Part model, mm, in its own coordinate system. Face numbers are marked on the shaded views. A direction names the side the tool comes from. Coordinates: 2 decimals unless noted, no trailing zeros. Loops run counter-clockwise (first coordinate to the right, second up) from the corner with the lowest first, then second, coordinate; pieces in that order, holes last. Notation, with made-up numbers: M 44.25,-3 L 51.25,-3 A24 cw 51.25,16 Z; hole C -8,56 d8. An arc over 180 degrees is marked long. Use CSV: the item, a comma, the result in double quotes. Start each with the question number.
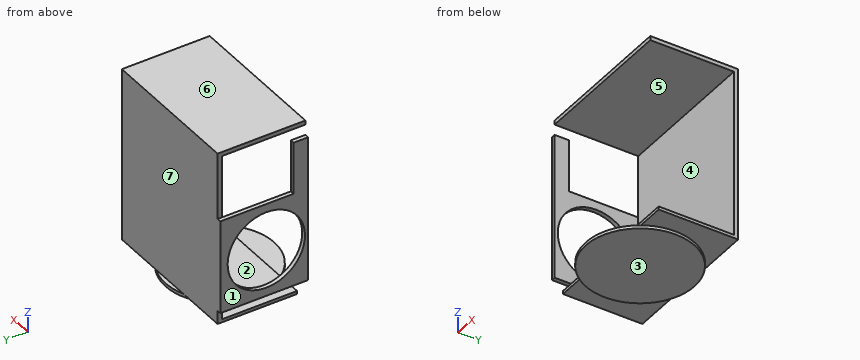
from build123d import *

# Parameters (mm, degrees)
SKETCH_1_R      = 26
EXTRUDE_1_DEPTH = 1.5
EXTRUDE_2_DEPTH = 1.5
SKETCH_3_W      = 70
SKETCH_3_H      = 2
EXTRUDE_3_DEPTH = 82
SKETCH_4_W      = 70
SKETCH_4_H      = 2
EXTRUDE_4_DEPTH = 40
SKETCH_5_R      = 18.5
EXTRUDE_5_DEPTH = 2


with BuildPart() as part:
    # 草图1 → 凸台-拉伸1 (new body)
    with BuildSketch(Plane.XY):
        Circle(SKETCH_1_R)
    extrude(amount=EXTRUDE_1_DEPTH)

    # 草图2 → 凸台-拉伸2 (add)
    with BuildSketch(Plane.XY.offset(1.5)):
        Polygon((-35, 24), (-35, -14), (-21.9089023, -14), (21.9089023, -14), (35, -14), (35, 24), align=None)
    extrude(amount=EXTRUDE_2_DEPTH)

    # 草图3 → 凸台-拉伸3 (add)
    with BuildSketch(Plane.XY.offset(3)):
        with Locations((0, 23)):
            Rectangle(SKETCH_3_W, SKETCH_3_H)
    extrude(amount=EXTRUDE_3_DEPTH)

    # 草图4 → 凸台-拉伸4 (add)
    with BuildSketch(Plane.XZ.offset(-22)):
        with Locations((0, 84)):
            Rectangle(SKETCH_4_W, SKETCH_4_H)
    extrude(amount=EXTRUDE_4_DEPTH)

    # 草图5 → 凸台-拉伸5 (add)
    with BuildSketch(Plane.ZY.offset(35)):
        Polygon((7.970689751, -18), (77.970689751, -18), (77.970689751, -11), (52.970689751, -11), (52.970689751, 22), (52.970689751, 24), (7.970689751, 24), (7.970689751, 22), align=None)
        with Locations((30.470689751, 2)):
            Circle(SKETCH_5_R, mode=Mode.SUBTRACT)
    extrude(amount=EXTRUDE_5_DEPTH)


solid = part.part
1. Slice it at C-C, the plane y = -4. List the corners of the cut face in (x, z), and give its area (3 significant figures).
2. Slice it at A-A, the plane z = 68.5. List the corners of the cut face in (x, y).
3. Slice it at B-B, the plane x = 24. List the corners of the cut face in (y, z), and give its area (3 significant figures).
4. Slice it at D-D, the plane z = 16. List the corners of the cut face in (x, y).
5. Pin check, flat tips, straight feed: pin 1 (6 mm diameter, centred on x = 4.5, z = 40.5, fed in from -Y); pin 2 (0.6 mm diameter, centred on x = -36.5, z = 69.5, fed in from +Y); pin 3 (1.6 mm diameter, centred on x = -7.5, z = 2, fed in from -Y). Stop position of each tip, or through.
6. Tool access for the marked faces 4, 5, 6 and 7: list every direction of +Z, -Z, +X, -X, +Y, -Y with a clear straight run to the whole face (end or side of a thin tool).
7. Wall check: probe 1 along Z at (x, y) = (16, 21); probe 2 along Z at (x, y) = (22.5, 10); probe 3 along X at (y, z) = (16, 15). Give the ranges that are in metal, low to high.
8. Two-plate mould, pull along Z, no slides. Class the marked faces 1, 2 and 3: pulls with the +Z half, pulls with the -Z half, needs draft (parallel to the pull), parting line crosses it, or undercut.
Found:
1,outline,"M -37,7.97 L -35,7.97 L -35,12.97 L -37,12.97 Z; M -37,47.97 L -35,47.97 L -35,52.97 L -37,52.97 Z; M -35,1.5 L -25.69,1.5 L -25.69,0 L 25.69,0 L 25.69,1.5 L 35,1.5 L 35,3 L -35,3 Z; M -35,83 L 35,83 L 35,85 L -35,85 Z"
1,area,"342 mm^2"
2,outline,"M -37,-18 L -35,-18 L -35,-11 L -37,-11 Z; M -35,22 L 35,22 L 35,24 L -35,24 Z"
3,outline,"M -18,83 L 22,83 L 22,3 L -14,3 L -14,1.5 L -10,1.5 L -10,0 L 10,0 L 10,1.5 L 24,1.5 L 24,85 L -18,85 Z"
3,area,"331 mm^2"
4,outline,"M -37,-18 L -35,-18 L -35,-9.53 L -37,-9.53 Z; M -37,13.53 L -35,13.53 L -35,22 L 35,22 L 35,24 L -37,24 Z"
5,pin 1,"y = 22"
5,pin 2,"y = -11"
5,pin 3,"y = -25.07"
6,face 4,"+X, -Y"
6,face 5,"+X, -X, -Y"
6,face 6,"+Z, +X, -X, +Y, -Y"
6,face 7,"+Z, +X, -X, +Y"
7,probe 1,"1.5 to 3, 83 to 85"
7,probe 2,"0 to 3, 83 to 85"
7,probe 3,"-37 to -35"
8,face 1,"needs draft"
8,face 2,"undercut"
8,face 3,"pulls with the -Z half"
